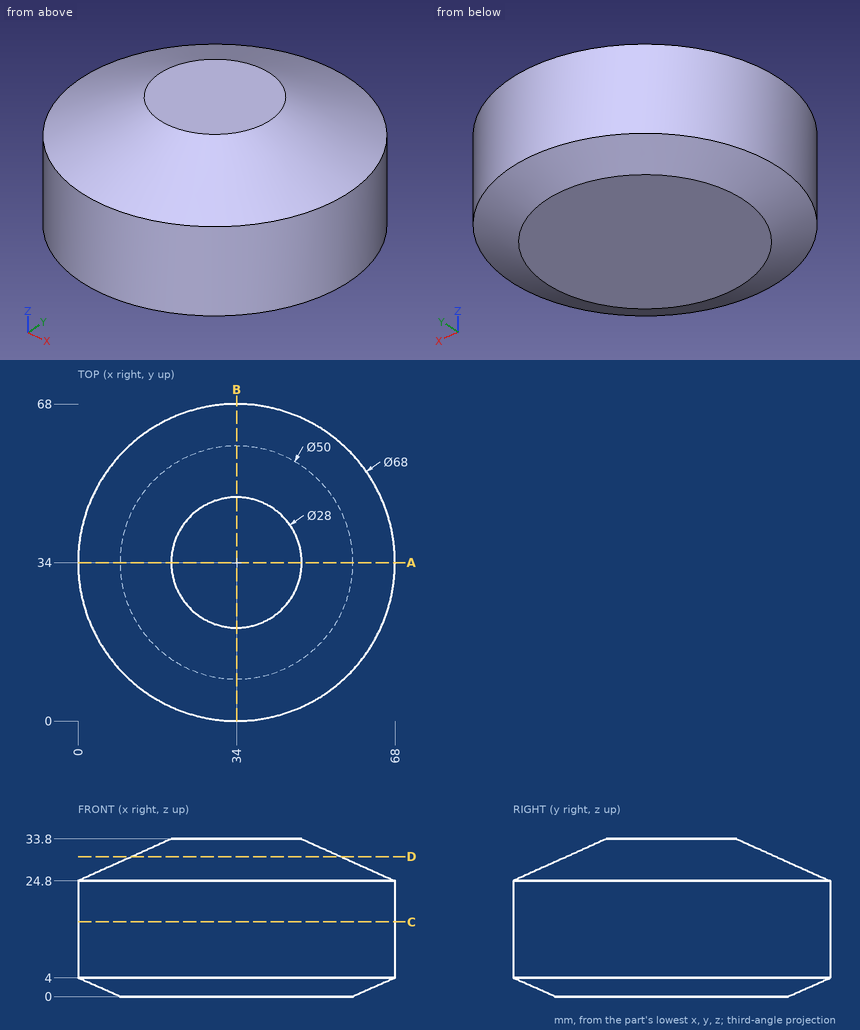
Verification items for this drawing (mm, ordinates from the low corner). Give positions to 0.01 mm unless a question says otherwise; leave off trailing zeros. Order: outer loops, then holes, each group sorted by start corner. A loop starts at its lowest first (then second) coordinate and runs counter-clockwise, first axis right, second up.
1) Cross-section at C-C (z = 16). Record the boundary of the cut face in (x, y).
Results are:
outline: circle Ø68 at (34, 34)
2) Cross-section at D-D (z = 30). Record the boundary of the cut face in (x, y), then the cut area to 3 significant figures.
Results are:
outline: circle Ø44.89 at (34, 34)
area: 1,580 mm2
3) Gauge pin test, flat ends, axial feed: pin 1 (4 mm diameter, centred on x = 49.5, y = 8.5, fed in from +Z); pin 2 (12 mm diameter, centred on x = 41, z = 30, fed in from +Y); pin 3 (3 mm diameter, centred on y = 37, z = 22, fed in from -X). Record the tip position at first contact, or that the pin passes through.
Results are:
pin 1: stops at z = 27.57
pin 2: stops at y = 67.76
pin 3: stops at x = 0.03
4) Material ranges on probe 1 along Y at (x, z) = (61.5, 12); probe 2 along Z at (x, y) = (51, 33.5); probe 3 along X at (y, z) = (60, 8.5), recorded low to high.
Results are:
probe 1: y = 14.01 to 53.99
probe 2: z = 0 to 32.45
probe 3: x = 12.09 to 55.91
5) Cross-section at A-A (y = 34). Record the boundary of the cut face in (x, z).
Results are:
outline: (0, 4) - (9, 0) - (59, 0) - (68, 4) - (68, 24.8) - (48, 33.8) - (20, 33.8) - (0, 24.8) - close
